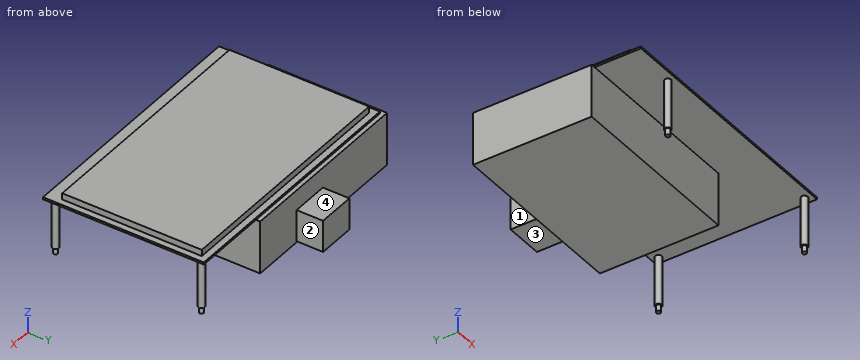
from build123d import *

# Parameters (mm, degrees)
F0_W      = 120.75
F0_H      = 75.9
F1_DEPTH  = 1
F2_W      = 114.75
F2_H      = 65.9
F3_DEPTH  = 3
F4_W      = 87
F4_H      = 56
F5_DEPTH  = 25
F6_W      = 18
F6_H      = 15
F7_DEPTH  = 12.5
F8_R      = 1.5
F9_DEPTH  = 23.5
F10_R     = 1
F11_DEPTH = 3


with BuildPart() as f1:
    # F0 (on Top) → F1 (new body)
    with BuildSketch(Plane.XY):
        with Locations((60.375, 37.95)):
            Rectangle(F0_W, F0_H)
    extrude(amount=F1_DEPTH)

    # F2 (on face) → F3 (join)
    with BuildSketch(Plane.XY.offset(1)):
        with Locations((60.375, 39.95)):
            Rectangle(F2_W, F2_H)
    extrude(amount=F3_DEPTH)

    # F4 (on face) → F5 (join)
    with BuildSketch(Plane(origin=(0, 0, 0), x_dir=(1, 0, 0), z_dir=(0, 0, -1))):
        with Locations((41.5, -49.9)):
            Rectangle(F4_W, F4_H)
    extrude(amount=F5_DEPTH)

    # F6 (on face) → F7 (join)
    with BuildSketch(Plane(origin=(0, 77.9, 0), x_dir=(-1, 0, 0), z_dir=(0, 1, 0))):
        with Locations((-51, -17)):
            Rectangle(F6_W, F6_H)
    extrude(amount=F7_DEPTH)

    # F8 (on face) → F9 (join)
    with BuildSketch(Plane(origin=(0, 0, 0), x_dir=(1, 0, 0), z_dir=(0, 0, -1))):
        with Locations((23.5, -3.5)):
            Circle(F8_R)
        with Locations((117.25, -3.5)):
            Circle(F8_R)
        with Locations((117.25, -72.4)):
            Circle(F8_R)
    extrude(amount=F9_DEPTH)

    # F10 (on face) → F11 (join)
    with BuildSketch(Plane(origin=(0, 0, -23.5), x_dir=(1, 0, 0), z_dir=(0, 0, -1))):
        with Locations((23.5, -3.5)):
            Circle(F10_R)
        with Locations((117.25, -3.5)):
            Circle(F10_R)
        with Locations((117.25, -72.4)):
            Circle(F10_R)
    extrude(amount=F11_DEPTH)


solid = f1.part
Input: part model. Units: mm. Frame: model coordinates. Face numbers are marked on the shaded views. A direction names the side the tool comes from. Coordinates: 2 decimals unless noted, no trailing zeros. Loops run counter-clockwise (first coordinate to the right, second up) from the corner with the lowest first, then second, coordinate; pieces in that order, holes last. Notation, with made-up numbers: (-19.75, -8.5) -> (-15.75, -8.5) arc R29 ccw to (-15.75, 13.5) -> close; hole circle Ø5 at (32, -6). An arc over 180 degrees is marked (long way). One line per item, written item: value.
(1) Cut plane C-C (y = 46.5). Output: boundary loops of the cut face in (x, z), then the cut area to 3 significant figures.
Answer below:
outline: (-2, -25) -> (85, -25) -> (85, 0) -> (120.75, 0) -> (120.75, 1) -> (117.75, 1) -> (117.75, 4) -> (3, 4) -> (3, 1) -> (0, 1) -> (0, 0) -> (-2, 0) -> close
area: 2,640 mm2
(2) Ray query, line 1 along Z through (x, y) = (60, 13); line 2 along Y through (x, z) = (44, -15); line 3 along Z through (x, y) = (10.5, 44). Return the intervals inside material, ascending.
Answer below:
line 1: z = 0 to 4
line 2: y = 21.9 to 90.4
line 3: z = -25 to 4
(3) Cut plane D-D (z = -17). Output: boundary loops of the cut face in (x, y), then the cut area to 3 significant figures.
Answer below:
outline: (-2, 21.9) -> (85, 21.9) -> (85, 77.9) -> (60, 77.9) -> (60, 90.4) -> (42, 90.4) -> (42, 77.9) -> (-2, 77.9) -> close; circle Ø3 at (23.5, 3.5); circle Ø3 at (117.25, 3.5); circle Ø3 at (117.25, 72.4)
area: 5,120 mm2
(4) Cut plane A-A (z = -2.5). Output: boundary loops of the cut face in (x, y), then the cut area to 3 significant figures.
Answer below:
outline: (-2, 21.9) -> (85, 21.9) -> (85, 77.9) -> (-2, 77.9) -> close; circle Ø3 at (23.5, 3.5); circle Ø3 at (117.25, 3.5); circle Ø3 at (117.25, 72.4)
area: 4,890 mm2
(5) Cut plane B-B (x = 97). Output: boundary loops of the cut face in (y, z), then the cut area to 3 significant figures.
Answer below:
outline: (0, 0) -> (75.9, 0) -> (75.9, 1) -> (72.9, 1) -> (72.9, 4) -> (7, 4) -> (7, 1) -> (0, 1) -> close
area: 274 mm2
(6) Set-up query: the marked faces 1, 2, 3 and 4. Return all of +Z, -Z, +X, -X, +Y, -Y with unobstructed straight access to the full face (end or side cutting, diameter ignored); none if empty.
Answer below:
face 1: +Z, -Z, -X, +Y
face 2: +Z, -Z, +X, +Y
face 3: -Z, +X, -X, +Y
face 4: +Z, +X, -X, +Y
(7) Pin query (flat end, axial travel): pin 1 Ø1.5 at (y, z) = (28.5, 2.5) entering from -X; pin 2 Ø2.5 at (y, z) = (47.5, 2.5) entering from +X; pin 3 Ø6 at (x, y) = (49, 85) entering from +Z; pin 4 Ø8 at (y, z) = (12.5, -20.5) entering from -X. Return the tip coordinate at first contact, or that it passes through.
Answer below:
pin 1: stops at x = 3
pin 2: stops at x = 117.75
pin 3: stops at z = -9.5
pin 4: passes through
